Autodesk Inventor part; units mm, degrees
ref_plane "YZ Plane" through (0, 0, 0) normal (1, 0, 0) x (0, 1, 0)
ref_plane "XZ Plane" through (0, 0, 0) normal (0, 1, 0) x (-1, 0, 0)
ref_plane "XY Plane" through (0, 0, 0) normal (0, 0, 1) x (1, 0, 0)
sketch "草圖1" plane through (0, 0, 0) normal (0, 0, 1) x (1, 0, 0)
  line L0 (0, -11.505) -> (0, 11.505) construction
  line L1 (2, -11.505) -> (2, 11.505)
  line L2 (-2, 11.505) -> (-2, -11.505)
  arc A0 (-2, -11.505) -> (2, -11.505) centre (0, -11.505) ccw
  arc A1 (2, 11.505) -> (-2, 11.505) centre (0, 11.505) ccw
  point P0 (0, 0)
  dimension "d0" = 23.01
  dimension "d1" = 4
extrude "擠出1" add sketch "草圖1" along normal blind 1
sketch "草圖2" plane through (0, 0, 1) normal (0, 0, 1) x (1, 0, 0)
  arc A0 (2, 11.505) -> (-2, 11.505) centre (0, 11.505) ccw
  circle A1 centre (0, 11.505) radius 0.75
  arc A2 (-2, -11.505) -> (2, -11.505) centre (0, -11.505) ccw
  circle A3 centre (0, -11.505) radius 0.75
  point P0 (0, 0)
  dimension "d4" = 1.5
  dimension "d5" = 1.5
extrude "擠出2" add sketch "草圖2" along normal blind 1
sketch "草圖3" plane through (0, 0, 1) normal (0, 0, 1) x (1, 0, 0)
  circle A0 centre (0, 11.505) radius 0.75
  circle A1 centre (0, -11.505) radius 0.75
  circle A2 centre (0, 11.505) radius 1
  circle A3 centre (0, -11.505) radius 1
  point P0 (0, 0)
  dimension "d8" = 2
  dimension "d9" = 2
extrude "擠出3" cut sketch "草圖3" along normal mid plane 10 contours A0 | A1 | A2 | A3
properties part number "連桿2"
Design review of the part built by this model. Coordinates are the model's own, in mm. Coordinates: 2 decimals unless noted, no trailing zeros. Write each loop counter-clockwise with the first axis right and the second up, starting at its lowest first coordinate (ties: lowest second). Pieces come first, ordered by that corner, then holes. Notation, with made-up numbers: (79.25, 3) - (127.25, 3) arc R20 ccw to (127.25, 41) - close; hole circle Ø3 at (83.5, 31). An arc over 180 degrees is marked (long way). Use one line per item in the form item = value.
Q1. The part is to be moulded in two halves that separate along Y. For faces 1 (the flat face through (0, 0, 0)), 2 (the cylindrical face through (0.044, -13.505, 0.493)), 3 (the cylindrical face through (-0.044, 13.505, 0.493)), 4 (the cylindrical face through (0.538, -10.662, 0.507)), say which applies: +Y half, -Y half, draft (parallel to the pull), parting line (faces both ways), or undercut.
Taken from the geometry:
face_1 = draft
face_2 = -Y half
face_3 = +Y half
face_4 = undercut
Q2. Consider section B-B (z = 0.15). Write out the cut boundary in (x, y) (3 decimals).
Taken from the geometry:
outline = (-2, -11.505) arc R2 ccw to (2, -11.505) - (2, 11.505) arc R2 ccw to (-2, 11.505) - close; hole circle Ø2 at (0, -11.505); hole circle Ø2 at (0, 11.505)
Q3. Consider section A-A (x = 0). Write out the cut boundary in (y, z) (3 decimals).
Taken from the geometry:
outline = (-13.505, 0) - (-12.505, 0) - (-12.505, 1) - (-13.505, 1) - close; (-10.505, 0) - (10.505, 0) - (10.505, 1) - (-10.505, 1) - close; (12.505, 0) - (13.505, 0) - (13.505, 1) - (12.505, 1) - close
Q4. For probe 1 along Y at (x, z) = (-0.1, 0.3); probe 2 along X at (y, z) = (-11, 0.15); probe 3 along Y at (x, z) = (0.75, 0.9), list the stretches that pass through material, from the lowest coordinate up.
Taken from the geometry:
probe_1 = -13.5 to -12.5, -10.51 to 10.51, 12.5 to 13.5
probe_2 = -2 to -0.86, 0.86 to 2
probe_3 = -13.36 to -12.17, -10.84 to 10.84, 12.17 to 13.36
Q5. Consider section C-C (x = 1.75). Write out the cut boundary in (y, z), plus the area to 3 significant figures.
Taken from the geometry:
outline = (-12.47, 0) - (12.47, 0) - (12.47, 1) - (-12.47, 1) - close
area = 24.9 mm^2
